```python
from build123d import *

# Parameters (mm, degrees)
SKETCH2_R                       = 1.4
BOSS_EXTRUDE1_DEPTH             = 14
BOSS_EXTRUDE2_REACH             = 34.049
BOSS_EXTRUDE2_END_RADIUS        = 107
SKETCH3_W                       = 14
SKETCH3_H                       = 14
BOSS_EXTRUDE2_DIRECTION_2_DEPTH = 3
SKETCH19_W                      = 15.846179349
SKETCH19_H                      = 3
CUT_EXTRUDE4_DEPTH              = 22
CUT_EXTRUDE8_DEPTH              = 34.788712692
SKETCH25_W                      = 10
SKETCH25_H                      = 3
CUT_EXTRUDE9_DEPTH              = 2
CUT_EXTRUDE10_DEPTH             = 0.2


with BuildPart() as part:
    # Sketch2 → Boss-Extrude1 (new body)
    with BuildSketch(Plane(origin=(0, 0, 0), x_dir=(1, 0, 0), z_dir=(0, 1, 0))):
        with BuildLine():
            ThreePointArc((-13.376751707, 9.244064366), (0, 8.25), (13.376751707, 9.244064366))
            ThreePointArc((13.376751707, 9.244064366), (22.755560222, 2.304111135), (15.815606991, -7.07469738))
            ThreePointArc((15.815606991, -7.07469738), (0, -8.25), (-15.815606991, -7.07469738))
            ThreePointArc((-15.815606991, -7.07469738), (-22.755560222, 2.304111135), (-13.376751707, 9.244064366))
        make_face()
        with Locations(Location((-14.596179349, 1.084683493, 0), (0, 0, 270))):
            Circle(SKETCH2_R, mode=Mode.SUBTRACT)
        with Locations(Location((14.596179349, 1.084683493, 0), (0, 0, 270))):
            Circle(SKETCH2_R, mode=Mode.SUBTRACT)
    extrude(amount=BOSS_EXTRUDE1_DEPTH)

    # Boss-Extrude2: up to this cylinder (the profile starts outside it)
    boss_extrude2_end = Plane(origin=(0, 7, -98.75), z_dir=(0, -1, 0)) * Cylinder(BOSS_EXTRUDE2_END_RADIUS, 283.098, mode=Mode.PRIVATE)
    # Sketch3 → Boss-Extrude2 (add, up to the surface)
    with BuildSketch(Plane.XY.offset(8.25), mode=Mode.PRIVATE) as boss_extrude2_sk1:
        with Locations((0, 7)):
            Rectangle(SKETCH3_W, SKETCH3_H)
    boss_extrude2_tool1 = extrude(boss_extrude2_sk1.sketch, amount=-BOSS_EXTRUDE2_REACH, mode=Mode.PRIVATE) - boss_extrude2_end
    add(boss_extrude2_tool1.solids().sort_by_distance((0, 7, 8.25))[0])
    add(boss_extrude2_tool1.solids().sort_by_distance((0, 7, 8.25))[1])

    # Sketch3 → Boss-Extrude2 direction 2 (add)
    with BuildSketch(Plane.XY.offset(8.25)):
        with Locations((0, 7)):
            Rectangle(SKETCH3_W, SKETCH3_H)
    extrude(amount=BOSS_EXTRUDE2_DIRECTION_2_DEPTH)

    # Sketch19 → Cut-Extrude4 (cut)
    with BuildSketch(Plane.XY.offset(8.25)):
        with Locations((-14.923089674, 7)):
            Rectangle(SKETCH19_W, SKETCH19_H)
    cut_extrude4 = extrude(amount=-CUT_EXTRUDE4_DEPTH, mode=Mode.SUBTRACT)

    # Mirror2: Cut-Extrude4 across plane
    add(cut_extrude4.mirror(Plane(origin=(0, 0, 0), x_dir=(0, 0, 1), z_dir=(1, 0, 0))), mode=Mode.SUBTRACT)

    # Sketch24 → Cut-Extrude8 (cut, through all)
    with BuildSketch(Plane.XY.offset(11.25)):
        Polygon((-5, 8.5), (-7, 8.5), (-7, 5.5), (-5, 5.5), (-5, 2), (5, 2), (5, 5.5), (7, 5.5), (7, 8.5), (5, 8.5), (5, 12), (-5, 12), align=None)
    extrude(amount=-CUT_EXTRUDE8_DEPTH, mode=Mode.SUBTRACT)


with BuildPart() as cut_extrude8_kept_piece:
    # of the separate pieces the step leaves, the one the design keeps (cut_extrude8_pieces_kept)
    add(part.part.solids().sort_by_distance((15.815606991, 0, 7.07469738))[0])

    # Sketch25 → Cut-Extrude9 (cut)
    with BuildSketch(Plane(origin=(0, 2, 0), x_dir=(1, 0, 0), z_dir=(0, 1, 0))):
        with Locations((0, 2.25)):
            Rectangle(SKETCH25_W, SKETCH25_H)
    extrude(amount=-CUT_EXTRUDE9_DEPTH, mode=Mode.SUBTRACT)

    # Sketch26 → Cut-Extrude10 (cut)
    with BuildSketch(Plane(origin=(0, 2, 0), x_dir=(1, 0, 0), z_dir=(0, 1, 0))):
        Polygon((-2.771713643, -4.706914557), (-1.224918771, -4.706914557), (-1.224918771, -5.032555583), (-2.486777746, -5.032555583), (-2.486777746, -6.00947866), (-1.224918771, -6.00947866), (-1.224918771, -6.335119685), (-2.486777746, -6.335119685), (-2.486777746, -7.881914557), (-2.771713643, -7.881914557), align=None)
        with BuildLine():
            add(Edge.make_bspline(
                [(-0.431168771, -7.393453019), (-0.413488364, -7.394503641), (-0.378827994, -7.396563264), (-0.328718213, -7.410693533), (-0.283365915, -7.435783889), (-0.242968807, -7.469223695), (-0.209670789, -7.509769047), (-0.18368627, -7.554759621), (-0.16967909, -7.605288923), (-0.16763447, -7.640150128), (-0.166585438, -7.658036352)],
                knots=[0, 0, 0, 0, 1.020151414, 1.999887582, 2.974338812, 3.990962822, 5.007586832, 5.987933904, 6.967670073, 8, 8, 8, 8], degree=3))
            add(Edge.make_bspline(
                [(-0.166585438, -7.658036352), (-0.167670019, -7.675492801), (-0.169808796, -7.709916663), (-0.183654162, -7.760064847), (-0.209868822, -7.805083538), (-0.242739137, -7.846179049), (-0.283375901, -7.879689696), (-0.328825433, -7.904566588), (-0.37871036, -7.919708598), (-0.413468739, -7.921637453), (-0.431168771, -7.922619685)],
                knots=[0, 0, 0, 0, 1.009421747, 1.99056486, 2.972319754, 3.999869655, 5.017953583, 5.993804169, 6.978383603, 8, 8, 8, 8], degree=3))
            add(Edge.make_bspline(
                [(-0.431168771, -7.922619685), (-0.448881557, -7.921672994), (-0.483461555, -7.919824803), (-0.533160278, -7.904255686), (-0.5788866, -7.879922976), (-0.619515453, -7.846116565), (-0.652661066, -7.805295007), (-0.677721235, -7.759754806), (-0.69277087, -7.710060216), (-0.69475014, -7.675521076), (-0.695752105, -7.658036352)],
                knots=[0, 0, 0, 0, 1.022052826, 1.995314843, 2.982371812, 4.00089066, 5.028879526, 6.005146991, 6.990147033, 8, 8, 8, 8], degree=3))
            add(Edge.make_bspline(
                [(-0.695752105, -7.658036352), (-0.694788629, -7.640120843), (-0.692907561, -7.605143011), (-0.67768964, -7.555069535), (-0.652855505, -7.509559594), (-0.619286325, -7.469285553), (-0.578896428, -7.435551358), (-0.533270585, -7.410999724), (-0.483341859, -7.396448778), (-0.448861415, -7.394468924), (-0.431168771, -7.393453019)],
                knots=[0, 0, 0, 0, 1.032775665, 2.016367738, 2.991239715, 4.008302682, 5.025365648, 6.011011707, 6.979408107, 8, 8, 8, 8], degree=3))
        make_face()
        with BuildLine():
            Line((0.647517126, -5.683837634), (0.362581229, -5.683837634))
            add(Edge.make_bspline(
                [(0.362581229, -5.683837634), (0.364438289, -5.646036186), (0.368085506, -5.571795148), (0.385165454, -5.463551318), (0.409604678, -5.360087322), (0.444159069, -5.2622339), (0.487072621, -5.16912584), (0.53853486, -5.081132968), (0.599489281, -4.998590961), (0.668619676, -4.922265011), (0.743702656, -4.852244857), (0.824715901, -4.79177903), (0.909846747, -4.740690856), (0.998836916, -4.697981444), (1.092690427, -4.665923155), (1.190555591, -4.642136382), (1.292862379, -4.627824983), (1.362567256, -4.626286663), (1.398017927, -4.625504301)],
                knots=[0, 0, 0, 0, 1.10065271, 2.161652631, 3.183658789, 4.190468796, 5.17591951, 6.163126047, 7.15150782, 8.156236427, 9.156009102, 10.134482811, 11.092018607, 12.041330605, 13.001268258, 13.972401359, 14.968799086, 16, 16, 16, 16], degree=3))
            add(Edge.make_bspline(
                [(1.398017927, -4.625504301), (1.432832323, -4.626319329), (1.501241367, -4.627920831), (1.601083338, -4.64167405), (1.696131312, -4.663214694), (1.7861995, -4.693436536), (1.870569287, -4.734062409), (1.949874478, -4.782864462), (2.025059213, -4.839306738), (2.092738224, -4.905758412), (2.154884839, -4.976699146), (2.208499027, -5.052434601), (2.254412397, -5.130656882), (2.292682649, -5.211962465), (2.320855004, -5.297116898), (2.342243807, -5.384880432), (2.354333675, -5.47616151), (2.356189167, -5.537943886), (2.357132511, -5.569354461)],
                knots=[0, 0, 0, 0, 1.111607364, 2.184268762, 3.212621178, 4.221274766, 5.211760367, 6.196651075, 7.1921475, 8.207485113, 9.220403448, 10.201281604, 11.166441695, 12.114753415, 13.065576456, 14.026450734, 14.996634279, 16, 16, 16, 16], degree=3))
            add(Edge.make_bspline(
                [(2.357132511, -5.569354461), (2.355596479, -5.613575711), (2.352551372, -5.701242191), (2.32650333, -5.830069959), (2.285821138, -5.954886846), (2.236837822, -6.055341399), (2.187423533, -6.136288925), (2.142894151, -6.202935536), (2.090765358, -6.274695497), (2.030278435, -6.35132851), (1.962684615, -6.433434831), (1.887371653, -6.52096486), (1.803802494, -6.613014251), (1.745147997, -6.675884332), (1.714754706, -6.708462033)],
                knots=[0, 0, 0, 0, 1.184426356, 2.348067706, 3.509069118, 4.696110526, 5.333549288, 6.050745305, 6.844228056, 7.710549037, 8.667450064, 9.695053472, 10.805634456, 12, 12, 12, 12], degree=3))
            Line((1.714754706, -6.708462033), (0.920368689, -7.556273532))
            Line((0.920368689, -7.556273532), (2.397837639, -7.556273532))
            Line((2.397837639, -7.556273532), (2.397837639, -7.881914557))
            Line((2.397837639, -7.881914557), (0.240465844, -7.881914557))
            Line((0.240465844, -7.881914557), (1.471795972, -6.567902137))
            add(Edge.make_bspline(
                [(1.471795972, -6.567902137), (1.501775127, -6.536607245), (1.559358947, -6.476496161), (1.64080457, -6.388736476), (1.713955653, -6.307320821), (1.779285716, -6.232403024), (1.835377539, -6.162887244), (1.885154492, -6.101024906), (1.925037564, -6.044097655), (1.968322244, -5.978111527), (2.010244927, -5.897546067), (2.046269707, -5.799090506), (2.068236034, -5.697737927), (2.070871135, -5.629246794), (2.072196613, -5.594795166)],
                knots=[0, 0, 0, 0, 1.329631726, 2.553950428, 3.673215718, 4.687767853, 5.603093632, 6.413772471, 7.123043292, 7.734684054, 8.834405432, 9.900288307, 10.943827018, 12, 12, 12, 12], degree=3))
            add(Edge.make_bspline(
                [(2.072196613, -5.594795166), (2.071619904, -5.573131326), (2.070483321, -5.530436058), (2.06045241, -5.467837976), (2.045293594, -5.407454181), (2.023571824, -5.349098934), (1.994899996, -5.293358949), (1.959999144, -5.240166378), (1.919731015, -5.188741388), (1.873148078, -5.140523753), (1.82197477, -5.096362945), (1.767914273, -5.057243239), (1.710718821, -5.024550617), (1.650629567, -4.997750445), (1.587814034, -4.976727064), (1.52215073, -4.962159638), (1.453821086, -4.953013385), (1.407163558, -4.951775886), (1.383389522, -4.951145326)],
                knots=[0, 0, 0, 0, 0.991446411, 1.95395049, 2.89581595, 3.838931463, 4.798493298, 5.75982156, 6.748411868, 7.785213223, 8.824556874, 9.840280684, 10.836137867, 11.835679398, 12.848801643, 13.863922112, 14.911575587, 16, 16, 16, 16], degree=3))
            add(Edge.make_bspline(
                [(1.383389522, -4.951145326), (1.358560267, -4.951793963), (1.309799709, -4.953067778), (1.238208872, -4.961978337), (1.169913916, -4.977350635), (1.104743047, -4.99837519), (1.042585994, -5.025098302), (0.98374504, -5.058382956), (0.928352276, -5.098100839), (0.876303573, -5.143131915), (0.828348392, -5.193267525), (0.78621444, -5.249156563), (0.749398942, -5.309778575), (0.717277708, -5.374969989), (0.69119219, -5.445322347), (0.671259403, -5.520585908), (0.655487049, -5.600433875), (0.650217891, -5.655574631), (0.647517126, -5.683837634)],
                knots=[0, 0, 0, 0, 1.031018746, 2.02475058, 2.990194455, 3.934040569, 4.864654155, 5.795059489, 6.735614925, 7.690564532, 8.649604399, 9.611025574, 10.590972636, 11.591080095, 12.624614302, 13.701020113, 14.821632451, 16, 16, 16, 16], degree=3))
        make_face()
    extrude(amount=-CUT_EXTRUDE10_DEPTH, mode=Mode.SUBTRACT)


solid = cut_extrude8_kept_piece.part
```
For this review, take the finished solid that the model builds, in its own axes (mm). A direction names the side the tool comes from. Coordinates: 2 decimals unless noted, no trailing zeros. Loops run counter-clockwise (first coordinate to the right, second up) from the corner with the lowest first, then second, coordinate; pieces in that order, holes last. Notation, with made-up numbers: (22, 38.5) -> (60, 38.5) arc R32 ccw to (60, 76.5) -> close; hole circle Ø6 at (-20, 84). An arc over 180 degrees is marked (long way). Return JSON: item names as keys, results as strings. Group by question number.
(1) Consider section C-C, the plane x = -15. Give the boundary of the cut face in (y, z), plus the area to 3 significant figures.
(2) To check wall thickness, follow L1, parallel to X at y = 4.75, z = 9.75; L2, parallel to X at y = 4.25, z = -5.25; L3, parallel to Z at x = 2.5, y = 0.45. State the ranges of each line that lie inside material, in increasing order.
(3) Consider section D-D, the plane z = 9.75. Give the boundary of the cut face in (x, y).
(4) Tool access review of faces 1 (the flat face through (0, 2, -6)), 2 (the flat face through (0, 1, -0.75)), 3 (the flat face through (-7, 3, 10)), 4 (the flat face through (-12, 5.5, -1)): name each direction out of +Z, -Z, +X, -X, +Y, -Y from which nothing blocks a thin tool from reaching the whole face with its end or side.
(5) Mouldability with a two-part tool opening along X and no side actions: class faces 5 (the flat face through (7, 3, 10)), 6 (the flat face through (12, 5.5, -1)), 7 (the cylindrical face through (-13.416, 2.712, -0.332)) as pulls with the +X half, pulls with the -X half, needs draft (parallel to the pull), parting line crosses it, or undercut.
(6) Consider section B-B, the plane z = -1.75. Give the boundary of the cut face in (x, y), plus the area to 3 significant figures.
(7) For pin 1 Ø1.6 at (y, z) = (3.5, 10) entering from -X; pin 2 Ø1 at (y, z) = (4, 3) entering from +X; pin 3 Ø1.7 at (x, z) = (-2, 5.5) entering from +Y; pin 4 Ø4.5 at (x, z) = (14.6, -1.08) entering from +Y, all flat-tipped, find the tip position at first contact; note any pin that passes through.
Results below:
{
 "1": {"outline": "(0, -9.32) -> (5.5, -9.32) -> (5.5, -2.43) -> (0, -2.43) -> close; (0, 0.26) -> (5.5, 0.26) -> (5.5, 7.19) -> (0, 7.19) -> close", "area": "76.1 mm2"},
 "2": {"L1": "x = -7 to -5, 5 to 7", "L2": "x = -21.72 to -5, 5 to 21.72", "L3": "z = -8.28 to -3.75, -0.75 to 11.25"},
 "3": {"outline": "(-7, 0) -> (7, 0) -> (7, 5.5) -> (5, 5.5) -> (5, 2) -> (-5, 2) -> (-5, 5.5) -> (-7, 5.5) -> close"},
 "4": {"face 1": "+Z, -Z, +Y", "face 2": "+Y, -Y", "face 3": "+Z, -X, +Y, -Y", "face 4": "+Z, -Z, +X, -X, +Y"},
 "5": {"face 5": "pulls with the +X half", "face 6": "needs draft", "face 7": "undercut"},
 "6": {"outline": "(-22.82, 0) -> (-15.83, 0) -> (-15.83, 5.5) -> (-22.82, 5.5) -> close; (-13.36, 0) -> (-5, 0) -> (-5, 5.5) -> (-13.36, 5.5) -> close; (5, 0) -> (13.36, 0) -> (13.36, 5.5) -> (5, 5.5) -> close; (15.83, 0) -> (22.82, 0) -> (22.82, 5.5) -> (15.83, 5.5) -> close", "area": "169 mm2"},
 "7": {"pin 1": "stops at x = -7", "pin 2": "stops at x = 22.03", "pin 3": "stops at y = 2", "pin 4": "stops at y = 5.5"}
}
